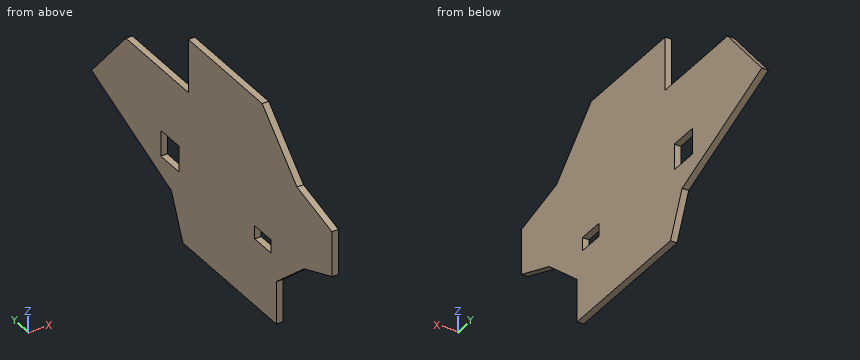
```python
from build123d import *

# Parameters (mm, degrees)
F1_W     = 12.621125
F1_H     = 6.403833
F1_W_2   = 14.245306
F1_H_2   = 12.555593
F0_DEPTH = 3.175


with BuildPart() as f0:
    # F1 (on Right) → F0 (new body)
    with BuildSketch(Plane.YZ):
        Polygon((-27.865971, 56.059395), (-54.780164, 30.102129), (-81.797782, 23.108517), (-81.797782, 1.158869), (-60.415494, -6.72708), (-38.755445, -24.869703), (-38.755445, -45.540605), (0.748058, -45.540605), (0.748058, 56.059395), align=None)
        with Locations((-28.339945, -9.928997)):
            Rectangle(F1_W, F1_H, mode=Mode.SUBTRACT)
        Polygon((29.362087, 56.059395), (0.748058, 56.059395), (0.748058, -45.540605), (12.285572, -45.540605), (33.50626, -45.540605), (42.517703, -24.869703), (104.240472, 0), (77.687405, 30.154637), (29.362087, 30.154637), align=None)
        with Locations((43.55493, -6.277797)):
            Rectangle(F1_W_2, F1_H_2, mode=Mode.SUBTRACT)
    extrude(amount=F0_DEPTH)


solid = f0.part
```
CAD build for the part. Positions are in the model's coordinates, mm. Coordinates: 2 decimals unless noted, no trailing zeros. Write each loop counter-clockwise with the first axis right and the second up, starting at its lowest first coordinate (ties: lowest second). Pieces come first, ordered by that corner, then holes. Notation, with made-up numbers: (-3.5, 71.25) -> (41.5, 71.25) arc R12 ccw to (41.5, 79.25) -> close; hole circle Ø3 at (-28.5, 87). An arc over 180 degrees is marked (long way). Use CSV: the item, a comma, the result in double quotes. Start each with the question number.
Item 1: Drop flat-ended pins along their axis: P1, Ø1.6, axis at x = 1.5, z = -36, coming from the -Y side; P2, Ø1.6, axis at x = 1, z = 44, coming from the +Y side; P3, Ø1, axis at x = 2, y = 47, coming from the -Z side. Give the stop position or say it passes through.
Item 2: Wall check: probe 1 along Y at (x, z) = (1.35, -8.5); probe 2 along Z at (x, y) = (1.3, -25.5); probe 3 along Z at (x, y) = (0.35, 33). Give the ranges that are in metal, low to high.
Item 3: Band-saw the part on C-C, the plane y = -32. Write the cut outline in (x, z) (3 decimals).
Item 4: Band-saw the part on D-D, the plane y = -64. Write the cut outline in (x, z) (3 decimals).
Item 5: Band-saw the part on A-A, the plane x = 1.4. Write the cut outline in (y, z), plus the area to 3 significant figures.
Item 6: Band-saw the part on B-B, the plane z = -9. Write the cut outline in (x, y) (1 decimal), plus the area to 3 significant figures.
Response values:
1,P1,"stops at y = -38.76"
1,P2,"stops at y = 29.36"
1,P3,"stops at z = -23.27"
2,probe 1,"y = -58.3 to -34.65, -22.03 to 36.43, 50.68 to 83.14"
2,probe 2,"z = -45.54 to -13.13, -6.73 to 56.06"
2,probe 3,"z = -45.54 to 30.15"
3,outline,"(0, -45.541) -> (3.175, -45.541) -> (3.175, -13.131) -> (0, -13.131) -> close; (0, -6.727) -> (3.175, -6.727) -> (3.175, 52.072) -> (0, 52.072) -> close"
4,outline,"(0, -5.405) -> (3.175, -5.405) -> (3.175, 27.716) -> (0, 27.716) -> close"
5,outline,"(-81.8, 1.16) -> (-60.42, -6.73) -> (-38.76, -24.87) -> (-38.76, -45.54) -> (33.51, -45.54) -> (42.52, -24.87) -> (104.24, 0) -> (77.69, 30.15) -> (29.36, 30.15) -> (29.36, 56.06) -> (-27.87, 56.06) -> (-54.78, 30.1) -> (-81.8, 23.11) -> close; hole (-34.65, -13.13) -> (-22.03, -13.13) -> (-22.03, -6.73) -> (-34.65, -6.73) -> close; hole (36.43, -12.56) -> (50.68, -12.56) -> (50.68, 0) -> (36.43, 0) -> close"
5,area,"11,500 mm2"
6,outline,"(0, -57.7) -> (3.2, -57.7) -> (3.2, -34.7) -> (0, -34.7) -> close; (0, -22) -> (3.2, -22) -> (3.2, 36.4) -> (0, 36.4) -> close; (0, 50.7) -> (3.2, 50.7) -> (3.2, 81.9) -> (0, 81.9) -> close"
6,area,"358 mm2"
